Autodesk Inventor part; units mm, degrees
ref_plane "Work Plane1" through (185, 0, 0) normal (1, 0, 0) x (0, 0, -1)
ref_plane "Work Plane2" through (20, 0, 0) normal (-1, 0, 0) x (0, 0, 1)
ref_plane "Work Plane3" through (102.5, 0, 0) normal (1, 0, 0) x (0, 0, -1)
sketch "Sketch1" plane through (0, 0, 0) normal (1, 0, 0) x (0, 1, 0)
  circle A0 centre (0, 0) radius 2.5
  dimension "d0" = 5
extrude "Extrusion1" add sketch "Sketch1" along normal blind 205
ref_plane "Work Plane1" through (185, 0, 0) normal (1, 0, 0) x (0, 0, -1)
sketch "Sketch2" plane through (185, 0, 0) normal (1, 0, 0) x (0, 0, -1)
  circle A0 centre (0, 0) radius 3
  dimension "d4" = 6
extrude "Extrusion2" add sketch "Sketch2" along normal blind 5
ref_plane "Work Plane2" through (20, 0, 0) normal (-1, 0, 0) x (0, 0, 1)
sketch "Sketch3" plane through (20, 0, 0) normal (-1, 0, 0) x (0, 0, 1)
  circle A0 centre (0, 0) radius 3
  dimension "d8" = 6
extrude "Extrusion3" add sketch "Sketch3" along normal blind 5
ref_plane "Work Plane3" through (102.5, 0, 0) normal (1, 0, 0) x (0, 0, -1)
sketch "Sketch4" plane through (102.5, 0, 0) normal (1, 0, 0) x (0, 0, -1)
  circle A0 centre (0, 0) radius 3
  dimension "d11" = 6
extrude "Extrusion4" add sketch "Sketch4" along normal mid plane 15
properties part number "roller stick"
Geometry: final body of the model. Coordinates: model frame, mm. A direction names the side the tool comes from. Round coordinates to 2 decimals unless told otherwise and drop trailing zeros. Write each loop counter-clockwise with the first axis right and the second up, starting at its lowest first coordinate (ties: lowest second). Pieces come first, ordered by that corner, then holes. Notation, with made-up numbers: M 85.5,-2.75 L 98.5,-2.75 A14 ccw 98.5,11.25 Z; hole C -40,-35.5 d1. An arc over 180 degrees is marked long. Write item = value, one per line.
Item 1: Section query A-A on y = 0. Return loops of the section in (x, z), then the cut area to 3 significant figures.
Findings:
outline = M 0,-2.5 L 15,-2.5 L 15,-3 L 20,-3 L 20,-2.5 L 95,-2.5 L 95,-3 L 110,-3 L 110,-2.5 L 185,-2.5 L 185,-3 L 190,-3 L 190,-2.5 L 205,-2.5 L 205,2.5 L 190,2.5 L 190,3 L 185,3 L 185,2.5 L 110,2.5 L 110,3 L 95,3 L 95,2.5 L 20,2.5 L 20,3 L 15,3 L 15,2.5 L 0,2.5 Z
area = 1,050 mm^2
Item 2: Material intervals for line 1 along Z through (x, y) = (60.5, -0.15); line 2 along Y through (x, z) = (164, -0.25); line 3 along Z through (x, y) = (174, 1.1) (3 decimals), sorted ascending. Write a range as [from, to].
Findings:
line_1 = [-2.5, 2.5]
line_2 = [-2.49, 2.49]
line_3 = [-2.245, 2.245]
Item 3: Pull-direction query (X, two-part tool) for faces 4 (the face through (110, 2, 2)), 5 (the face through (205, 0, 0)), 6 (the face through (187, 0, 3)); classes: pulls with the +X half, pulls with the -X half, needs draft (parallel to the pull), parting line crosses it, or undercut.
Findings:
face_4 = undercut
face_5 = pulls with the +X half
face_6 = needs draft
Item 4: Section query C-C on x = 119. Return loops of the section in (y, z).
Findings:
outline = C 0,0 d5
Item 5: Pin query (flat end, axial travel): P1, Ø1.5, axis at x = 62.5, y = -2.5, coming from the -Z side; P2, Ø1.5, axis at x = 166, y = 1, coming from the +Z side; P3, Ø3, axis at x = 69.5, z = 0.5, coming from the +Y side. Return the tip coordinate at first contact, or that it passes through.
Findings:
P1 = -1.79
P2 = 2.49
P3 = 2.5
Item 6: Access query for faces 1 (the face through (7.4, -0.54, 2.44)), 2 (the face through (190, 2, 2)), 3 (the face through (20, 2, -2)). Directions: +Z, -Z, +X, -X, +Y, -Y. A direction counts if a zero-diameter tool reaches every point of the face in a straight line with its end or side. Return the directions, or none.
Findings:
face_1 = -X
face_2 = +X
face_3 = none
